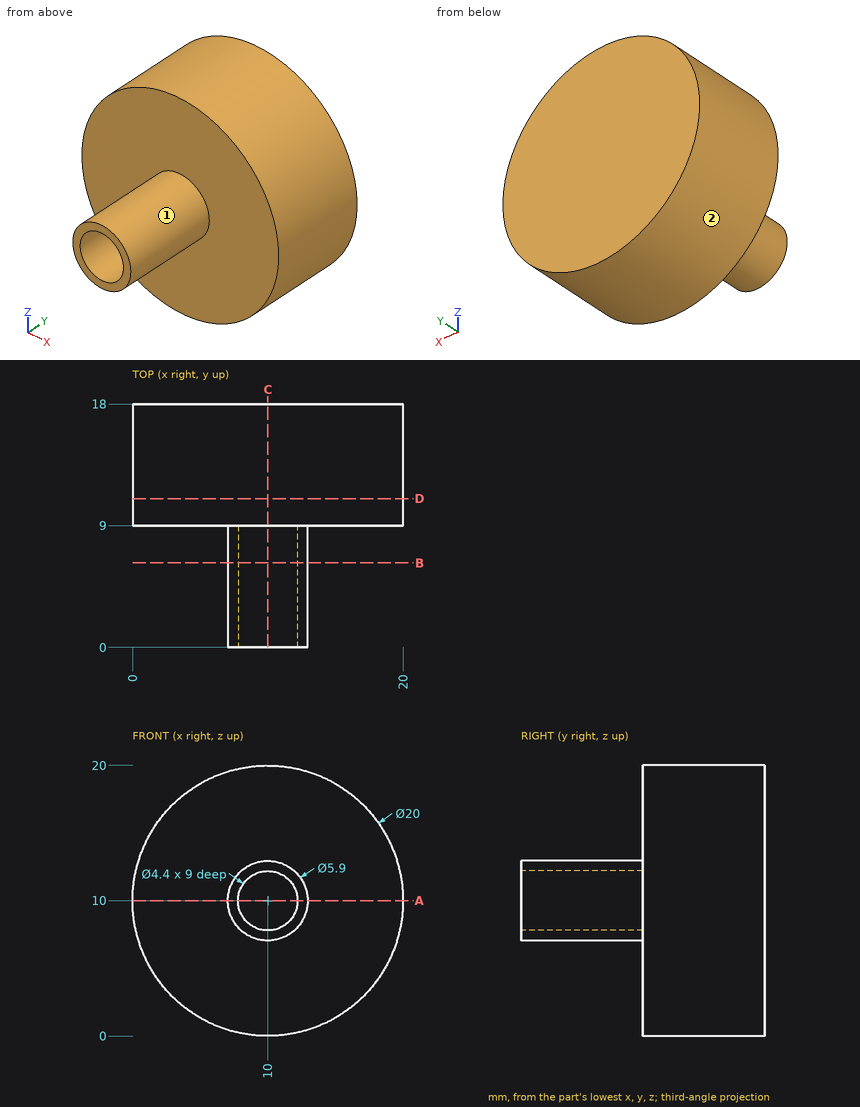
For this review, use the dimensioned drawing (mm, ordinates from the lowest corner) and the shaded views. A direction names the side the tool comes from. Round coordinates to 2 decimals unless told otherwise and drop trailing zeros. Write each loop counter-clockwise with the first axis right and the second up, starting at its lowest first coordinate (ties: lowest second). Pieces come first, ordered by that corner, then holes. Notation, with made-up numbers: (64.5, -24) - (102.5, -24) arc R18 cw to (102.5, 7) - close; hole circle Ø5 at (14.5, -13.5). An arc over 180 degrees is marked (long way). Answer as CSV lines item,"result". Start each with the question number.
(1) For pin 1 Ø4 at (y, z) = (6.5, 16) entering from -X; pin 2 Ø1.5 at (y, z) = (3.5, 11.5) entering from -X; pin 3 Ø4 at (x, z) = (10, 10) entering from -Y, all flat-tipped, find the tip position at first contact; note any pin that passes through.
(2) We need section A-A on z = 10. State the section outline as (x, y) points, plus the area to 4 significant figures.
(3) For the marked faces 1 and 2, list the 3-axis set-ups (+Z, -Z, +X, -X, +Y, -Y) from which the entire face can be reached by the end or side of a thin tool; tool diameter is ignored.
(4) We need section D-D on y = 11. State the section outline as (x, z) points.
(5) We need section B-B on y = 6.25. State the section outline as (x, z) points, plus the area to 3 significant figures.
(6) We need section C-C on x = 10. State the section outline as (y, z) points.
(7) To check wall thickness, follow line 1 (X direction, y = 3.25, z = 10); line 2 (Y direction, x = 9.25, z = 9.5). State the ranges of each line that lie inside material, in increasing order.
Worked answers:
1,pin 1,"through"
1,pin 2,"x = 7.15"
1,pin 3,"y = 9"
2,outline,"(0, 9) - (7.05, 9) - (7.05, 0) - (7.8, 0) - (7.8, 9) - (12.2, 9) - (12.2, 0) - (12.95, 0) - (12.95, 9) - (20, 9) - (20, 18) - (0, 18) - close"
2,area,"193.5 mm²"
3,face 1,"-Y"
3,face 2,"+Y, -Y"
4,outline,"circle Ø20 at (10, 10)"
5,outline,"circle Ø5.9 at (10, 10); hole circle Ø4.4 at (10, 10)"
5,area,"12.1 mm²"
6,outline,"(0, 7.05) - (9, 7.05) - (9, 0) - (18, 0) - (18, 20) - (9, 20) - (9, 12.95) - (0, 12.95) - (0, 12.2) - (9, 12.2) - (9, 7.8) - (0, 7.8) - close"
7,line 1,"7.05 to 7.8, 12.2 to 12.95"
7,line 2,"9 to 18"
